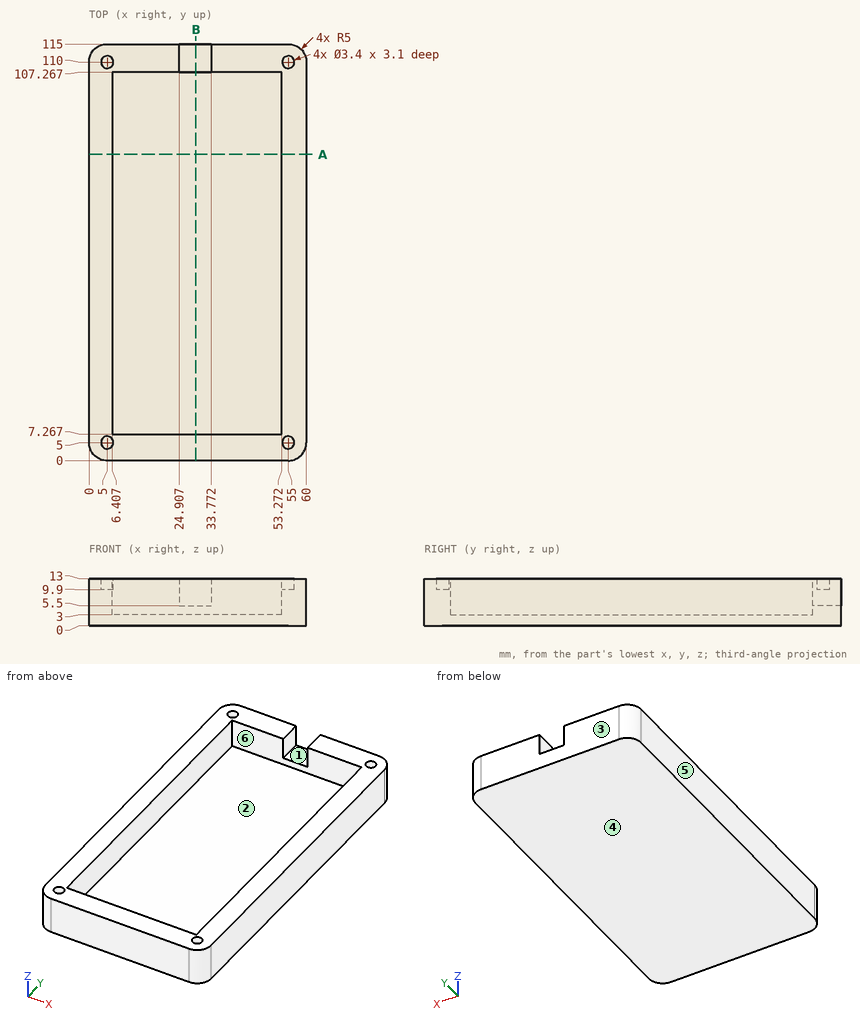
Job drawing, mm, ordinate dimensions from the low corner. One solid piece. A direction names the side the tool comes from. Coordinates: 2 decimals unless noted, no trailing zeros. Write each loop counter-clockwise with the first axis right and the second up, starting at its lowest first coordinate (ties: lowest second). Pieces come first, ordered by that corner, then holes. Notation, with made-up numbers: (-27.75, 51) - (17.25, 51) arc R24 cw to (17.25, 69) - close; hole circle Ø1 at (-35.5, 83.25). An arc over 180 degrees is marked (long way). Use a Markdown table: item, result. Add a question column.
Item 1: 3-axis set-ups, long thin cutter, end or side, ignore diameter. For the marked faces 1, 2 and 3: which of +Z, -Z, +X, -X, +Y, -Y reach the whole face in a straight line?
Item 2: Drill centre lines: L1, parallel to Y at x = 55, z = 11.1; L2, parallel to X at y = 67.5, z = 5; L3, parallel to Y at x = 51, z = 7.5. Where is each one in solid material? Low to high. Write a range as from..to.
Item 3: Mould opens along X. For the marked faces 4, 5 and 6 say: pulls with the +X half, pulls with the -X half, needs draft (parallel to the pull), parting line crosses it, or undercut.
Item 4: Band-saw the part on B-B, the plane x = 29.5. Give the cut face in (y, z).
Item 5: Band-saw the part on A-A, the plane y = 84.5. Give the cut face in (x, z), and give its area (3 significant figures).
Item 6: Flat gauge pins, fed straight in: pin 1 (6 mm diameter, centred on x = 28.5, y = 113, fed in from +Z); pin 2 (2.5 mm diameter, centred on x = 55, y = 110, fed in from +Z); pin 3 (4 mm diameter, centred on y = 112.5, z = 10.5, fed in from +X) (3 decimals). Where does each tip first touch, or does it go through?
Numbers:
| question | item | result |
|---|---|---|
| 1 | face 1 | +Z, +Y |
| 1 | face 2 | +Z |
| 1 | face 3 | +Z, -Z, +X, -X, +Y |
| 2 | L1 | 0..3.3, 6.7..108.3, 111.7..115 |
| 2 | L2 | 0..6.41, 53.27..60 |
| 2 | L3 | 0..7.27, 107.27..115 |
| 3 | face 4 | needs draft |
| 3 | face 5 | pulls with the -X half |
| 3 | face 6 | undercut |
| 4 | outline | (0, 0) - (115, 0) - (115, 5.5) - (107.27, 5.5) - (107.27, 3) - (7.27, 3) - (7.27, 13) - (0, 13) - close |
| 5 | outline | (0, 0) - (60, 0) - (60, 13) - (53.27, 13) - (53.27, 3) - (6.41, 3) - (6.41, 13) - (0, 13) - close |
| 5 | area | 311 mm2 |
| 6 | pin 1 | z = 5.5 |
| 6 | pin 2 | z = 9.9 |
| 6 | pin 3 | x = 59.975 |
